Build history of the part. All positions in model axes, mm. Face numbers are marked on the shaded views. A direction names the side the tool comes from. Round coordinates to 2 decimals unless told otherwise and drop trailing zeros. Write each loop counter-clockwise with the first axis right and the second up, starting at its lowest first coordinate (ties: lowest second). Pieces come first, ordered by that corner, then holes. Notation, with made-up numbers: (-22.75, 72) -> (-2.75, 72) arc R35 cw to (-2.75, 104) -> close; hole circle Ø7 at (33, 74). An arc over 180 degrees is marked (long way). Answer in a Markdown table with one row per item.
```python
from build123d import *

# Parameters (mm, degrees)
SKETCH1_R           = 2.159
BOSS_EXTRUDE1_DEPTH = 2.54
SKETCH2_W           = 8.89
SKETCH2_H           = 6.35
BOSS_EXTRUDE2_DEPTH = 1.651
SKETCH3_W           = 8.89
SKETCH3_H           = 6.35
BOSS_EXTRUDE3_DEPTH = 1.651
SKETCH4_R           = 1.4605
CUT_EXTRUDE1_DEPTH  = 6.842
FILLET1_R           = 1.27


with BuildPart() as part:
    # Sketch1 → Boss-Extrude1 (new body)
    with BuildSketch(Plane(origin=(0, 0, 0), x_dir=(1, 0, 0), z_dir=(0, 1, 0))):
        Circle(SKETCH1_R)
    extrude(amount=BOSS_EXTRUDE1_DEPTH)

    # Sketch2 → Boss-Extrude2 (add)
    with BuildSketch(Plane(origin=(0, 2.54, 0), x_dir=(1, 0, 0), z_dir=(0, 1, 0))):
        Rectangle(SKETCH2_W, SKETCH2_H)
    extrude(amount=BOSS_EXTRUDE2_DEPTH)

    # Sketch3 → Boss-Extrude3 (add)
    with BuildSketch(Plane(origin=(0, 0, 0), x_dir=(-1, 0, 0), z_dir=(0, -1, 0))):
        Rectangle(SKETCH3_W, SKETCH3_H)
    extrude(amount=BOSS_EXTRUDE3_DEPTH)

    # Sketch4 → Cut-Extrude1 (cut, through all)
    with BuildSketch(Plane(origin=(0, 4.191, 0), x_dir=(1, 0, 0), z_dir=(0, 1, 0))):
        Circle(SKETCH4_R)
    extrude(amount=-CUT_EXTRUDE1_DEPTH, mode=Mode.SUBTRACT)

    # Fillet1
    fillet1_edges = [part.edges().sort_by_distance(p)[0] for p in [
        (-4.445, -0.8255, 3.175),
        (-4.445, -0.8255, -3.175),
        (4.445, -0.8255, -3.175),
        (4.445, -0.8255, 3.175),
        (4.445, 3.3655, 3.175),
        (4.445, 3.3655, -3.175),
        (-4.445, 3.3655, -3.175),
        (-4.445, 3.3655, 3.175),
    ]]
    fillet(fillet1_edges, radius=FILLET1_R)


solid = part.part
```
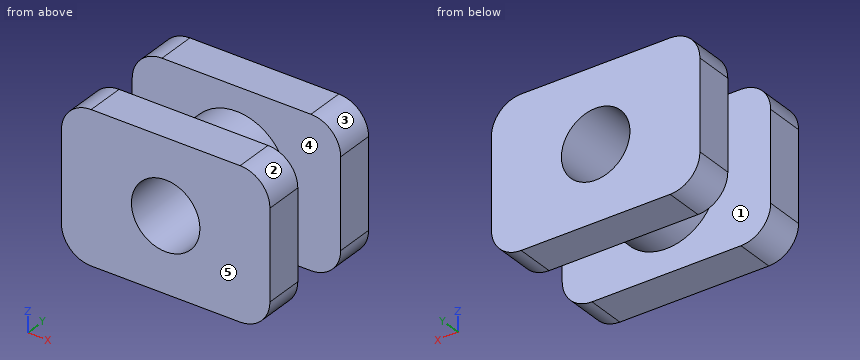
Q1. Wall check: line 1 (Z direction, x = 0, y = -1.05) (1 decimal); line 2 (Y direction, x = 4.25, z = -2.25); line 3 (Z direction, x = 0, y = 1.85). Give the ranges that are in metal, low to high. Write a range as [from, to].
A:
| item | result |
|---|---|
| line 1 | [-3.2, -1.5], [1.5, 3.2] |
| line 2 | [-1.65, 0], [2.54, 4.19] |
| line 3 | [-2.16, -1.46], [1.46, 2.16] |
Q2. Two-plate mould, pull along Y, no slides. Class the marked faces 3, 4 and 5: released by +Y, released by -Y, zero draft, split by the parting line, or undercut.
A:
| item | result |
|---|---|
| face 3 | zero draft |
| face 4 | undercut |
| face 5 | released by -Y |
Q3. Saw through at B-B on x = 2.75. Write the cut outline in (y, z) (3 decimals).
A:
| item | result |
|---|---|
| outline | (-1.651, -3.175) -> (0, -3.175) -> (0, 3.175) -> (-1.651, 3.175) -> close; (2.54, -3.175) -> (4.191, -3.175) -> (4.191, 3.175) -> (2.54, 3.175) -> close |
Q4. Saw through at D-D on x = 0. Write the cut outline in (y, z) (1 decimal).
A:
| item | result |
|---|---|
| outline | (-1.7, -3.2) -> (0, -3.2) -> (0, -2.2) -> (2.5, -2.2) -> (2.5, -3.2) -> (4.2, -3.2) -> (4.2, -1.5) -> (-1.7, -1.5) -> close; (-1.7, 1.5) -> (4.2, 1.5) -> (4.2, 3.2) -> (2.5, 3.2) -> (2.5, 2.2) -> (0, 2.2) -> (0, 3.2) -> (-1.7, 3.2) -> close |
Q5. Drop flat-ended pins along their axis: P1, Ø2, axis at x = 2, y = 1.5, coming from the +Z side; P2, Ø2.5, axis at x = 0, z = 0, coming from the -Y side. Give the stop position or say it passes through.
A:
| item | result |
|---|---|
| P1 | z = 1.91 |
| P2 | through |
Q6. Saw through at C-C on y = -0.3. Write the cut outline in (x, z) (1 decimal), plus the area to 3 significant figures.
A:
| item | result |
|---|---|
| outline | (-4.4, -1.9) arc R1.3 ccw to (-3.2, -3.2) -> (3.2, -3.2) arc R1.3 ccw to (4.4, -1.9) -> (4.4, 1.9) arc R1.3 ccw to (3.2, 3.2) -> (-3.2, 3.2) arc R1.3 ccw to (-4.4, 1.9) -> close; hole circle Ø2.9 at (0, 0) |
| area | 48.4 mm² |
Q7. Saw through at A-A on z = 0. Write the cut outline in (x, y) (1 decimal).
A:
| item | result |
|---|---|
| outline | (-4.4, -1.7) -> (-1.5, -1.7) -> (-1.5, 4.2) -> (-4.4, 4.2) -> (-4.4, 2.5) -> (-2.2, 2.5) -> (-2.2, 0) -> (-4.4, 0) -> close; (1.5, -1.7) -> (4.4, -1.7) -> (4.4, 0) -> (2.2, 0) -> (2.2, 2.5) -> (4.4, 2.5) -> (4.4, 4.2) -> (1.5, 4.2) -> close |
Q8. Which spindle directions (+Z, -Z, +X, -X, +Y, -Y) get a long thin tool onto all of the face, cutting with end or side? Do the marked faces 1 and 2. Say none if no direction does.
A:
| item | result |
|---|---|
| face 1 | none |
| face 2 | +Z, +X, +Y, -Y |
